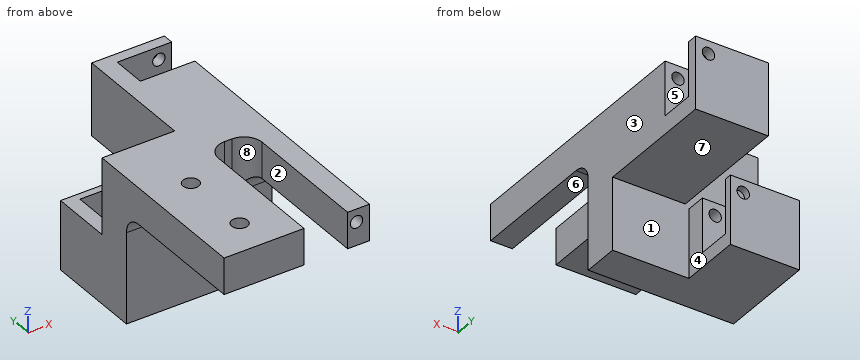
```python
from build123d import *

# Parameters (mm, degrees)
SKETCH1_W               = 40
SKETCH1_H               = 50
BOSS_EXTRUDE1_DEPTH     = 10
SKETCH2_W               = 40
SKETCH2_H               = 10
BOSS_EXTRUDE2_DEPTH     = 30
SKETCH3_W               = 20
SKETCH3_H               = 20
BOSS_EXTRUDE3_DEPTH     = 34
SKETCH4_W               = 19
SKETCH4_H               = 19
BOSS_EXTRUDE4_DEPTH     = 17
CUT_EXTRUDE4_DEPTH      = 9.5
CUT_EXTRUDE13_DEPTH     = 9.5
CUT_EXTRUDE7_DEPTH      = 93.694591653
CUT_EXTRUDE7_DEPTH_BACK = 3
SKETCH10_R              = 1.7
CUT_EXTRUDE9_REACH      = 74.328
SKETCH12_W              = 12
SKETCH12_H              = 40
FILLET2_R               = 5
CUT_EXTRUDE10_REACH     = 74.328
SKETCH13_R              = 2.2
SKETCH14_R              = 1.7
CUT_EXTRUDE14_DEPTH     = 20


with BuildPart() as part:
    # Sketch1 → Boss-Extrude1 (new body)
    with BuildSketch(Plane.XY):
        with Locations((13.634614932, -25)):
            Rectangle(SKETCH1_W, SKETCH1_H)
    extrude(amount=BOSS_EXTRUDE1_DEPTH)

    # Sketch2 → Boss-Extrude2 (add)
    with BuildSketch(Plane.XY):
        with Locations((13.634614932, -5)):
            Rectangle(SKETCH2_W, SKETCH2_H)
    extrude(amount=-BOSS_EXTRUDE2_DEPTH)

    # Sketch3 → Boss-Extrude3 (add)
    with BuildSketch(Plane(origin=(0, 0, 0), x_dir=(1, 0, 0), z_dir=(0, 1, 0))):
        with Locations((23.634614932, 0)):
            Rectangle(SKETCH3_W, SKETCH3_H)
    extrude(amount=BOSS_EXTRUDE3_DEPTH)

    # Sketch4 → Boss-Extrude4 (add)
    with BuildSketch(Plane(origin=(0, 0, 0), x_dir=(1, 0, 0), z_dir=(0, 1, 0))):
        with Locations((3.134614932, 20.5)):
            Rectangle(SKETCH4_W, SKETCH4_H)
    extrude(amount=BOSS_EXTRUDE4_DEPTH)

    # Sketch6 → Cut-Extrude4 (cut)
    with BuildSketch(Plane(origin=(0, 31, 0), x_dir=(1, 0, 0), z_dir=(0, 1, 0))):
        with BuildLine():
            Line((33.634614932, 5), (33.634614932, -10))
            Line((33.634614932, -10), (18.634614932, -10))
            ThreePointArc((18.634614932, -10), (23.028013215, 0.606601718), (33.634614932, 5))
        make_face()
    extrude(amount=-CUT_EXTRUDE4_DEPTH, mode=Mode.SUBTRACT)

    # Sketch7 → Cut-Extrude13 (cut)
    with BuildSketch(Plane(origin=(0, 15, 0), x_dir=(1, 0, 0), z_dir=(0, 1, 0))):
        with BuildLine():
            Line((-2.365385068, 11), (12.634614932, 11))
            Line((12.634614932, 11), (12.634614932, 26))
            ThreePointArc((12.634614932, 26), (2.028013215, 21.606601718), (-2.365385068, 11))
        make_face()
    extrude(amount=-CUT_EXTRUDE13_DEPTH, mode=Mode.SUBTRACT)

    # Sketch10 → Cut-Extrude7 (cut, two sides: drawn at the far end of the back side and taken through both)
    with BuildSketch(Plane(origin=(0, 31, 0), x_dir=(-1, 0, 0), z_dir=(0, -1, 0)).offset(-CUT_EXTRUDE7_DEPTH_BACK)):
        with Locations(Location((-30.099081026, -6.464466094, 0), (0, 0, 180))):
            Circle(SKETCH10_R)
    extrude(amount=CUT_EXTRUDE7_DEPTH + CUT_EXTRUDE7_DEPTH_BACK, mode=Mode.SUBTRACT)

    # Sketch12 → Cut-Extrude9 (cut, up to next)
    with BuildSketch(Plane.XY.offset(10), mode=Mode.PRIVATE) as cut_extrude9_sk1:
        with Locations((21.634614932, -30)):
            Rectangle(SKETCH12_W, SKETCH12_H)
    cut_extrude9_tool1 = extrude(cut_extrude9_sk1.sketch, amount=-CUT_EXTRUDE9_REACH, mode=Mode.PRIVATE) & part.part
    add(cut_extrude9_tool1.solids().sort_by_distance((21.634615, -30, 10))[0], mode=Mode.SUBTRACT)

    # Fillet2
    fillet2_edges = [part.edges().sort_by_distance(p)[0] for p in [
        (4.634614932, -10, 0),
        (30.634614932, -10, 0),
        (27.634614932, -10, 5),
        (15.634614932, -10, 5),
    ]]
    fillet(fillet2_edges, radius=FILLET2_R)

    # Sketch13 → Cut-Extrude10 (cut, up to next)
    with BuildSketch(Plane.XY.offset(10), mode=Mode.PRIVATE) as cut_extrude10_sk1:
        with Locations((4.634614932, -20)):
            Circle(SKETCH13_R)
    cut_extrude10_tool1 = extrude(cut_extrude10_sk1.sketch, amount=-CUT_EXTRUDE10_REACH, mode=Mode.PRIVATE) & part.part
    # Sketch13 → Cut-Extrude10 (cut, up to next)
    with BuildSketch(Plane.XY.offset(10), mode=Mode.PRIVATE) as cut_extrude10_sk2:
        with Locations((4.634614932, -40)):
            Circle(SKETCH13_R)
    cut_extrude10_tool2 = extrude(cut_extrude10_sk2.sketch, amount=-CUT_EXTRUDE10_REACH, mode=Mode.PRIVATE) & part.part
    add(cut_extrude10_tool1.solids().sort_by_distance((4.634615, -20, 10))[0], mode=Mode.SUBTRACT)
    add(cut_extrude10_tool2.solids().sort_by_distance((4.634615, -40, 10))[0], mode=Mode.SUBTRACT)

    # Sketch14 → Cut-Extrude14 (cut)
    with BuildSketch(Plane(origin=(0, 17, 0), x_dir=(1, 0, 0), z_dir=(0, 1, 0))):
        with Locations(Location((9.099081026, 14.535533906, 0), (0, 0, 180))):
            Circle(SKETCH14_R)
    extrude(amount=-CUT_EXTRUDE14_DEPTH, mode=Mode.SUBTRACT)


solid = part.part
```
The model under review builds one solid part; all positions refer to its coordinate system, in mm. Face numbers are marked on the shaded views. A direction names the side the tool comes from. Coordinates: 2 decimals unless noted, no trailing zeros. Order: outer loops, then holes, each group sorted by start corner. A loop starts at its lowest first (then second) coordinate and runs counter-clockwise, first axis right, second up. Notation, with made-up numbers: (-33.5, 74) -> (23.5, 74) arc R25 cw to (23.5, 97) -> close; hole circle Ø2 at (26, 59.25). An arc over 180 degrees is marked (long way). Answer in a Markdown table with one row per item. Add a question column.
Item 1: We need section B-B on y = -20. Write out the cut boundary in (x, z).
Item 2: To check wall thickness, follow probe 1 along X at (y, z) = (-27, 5.5); probe 2 along Y at (x, z) = (10, -24.5); probe 3 along Y at (x, z) = (28.5, 8). State the ranges of each line that lie inside material, in increasing order.
Item 3: We need section A-A on y = -34. Write out the cut boundary in (x, z).
Item 4: We need section C-C on x = 9.5. Write out the cut boundary in (y, z), plus the area to 3 significant figures.
Item 5: We need section D-D on z = 2.5. Write out the cut boundary in (x, y).
Item 6: Clearance check with flat-ended pins moving along their axes: pin 1 (5.5 mm diameter, centred on x = -1, z = -19.5, fed in from +Y); pin 2 (10 mm diameter, centred on x = 13, y = -36.5, fed in from -Z); pin 3 (2.5 mm diameter, centred on x = 9, z = -14.5, fed in from +Y); pin 4 (3.5 mm diameter, centred on x = 4.63, y = -20, fed in from +Z). State where each tip first meets the part, or that it passes through.
Item 7: Mouldability with a two-part tool opening along X and no side actions: class the marked faces 1, 2 and 3 as +X half, -X half, draft (parallel to the pull), parting line (faces both ways), or undercut.
Item 8: Machinability: for the marked faces 4, 5, 6, 7 and 8, which of the approach directions +Z, -Z, +X, -X, +Y, -Y give a long, thin tool a straight path to every point of the face, cutting with its end or side? Answer none if there is none.
Final values:
| question | item | result |
|---|---|---|
| 1 | outline | (-6.37, 0) -> (2.43, 0) -> (2.43, 10) -> (-6.37, 10) -> close; (6.83, 0) -> (15.63, 0) -> (15.63, 10) -> (6.83, 10) -> close; (27.63, 0) -> (33.63, 0) -> (33.63, 10) -> (27.63, 10) -> close; hole circle Ø3.4 at (30.1, 6.46) |
| 2 | probe 1 | x = -6.37 to 15.63, 27.63 to 28.7, 31.5 to 33.63 |
| 2 | probe 2 | y = -10 to 5.5, 15 to 17 |
| 2 | probe 3 | y = -50 to 21.5, 31 to 34 |
| 3 | outline | (-6.37, 0) -> (15.63, 0) -> (15.63, 10) -> (-6.37, 10) -> close; (27.63, 0) -> (33.63, 0) -> (33.63, 10) -> (27.63, 10) -> close; hole circle Ø3.4 at (30.1, 6.46) |
| 4 | outline | (-50, 0) -> (-15, 0) arc R5 cw to (-10, -5) -> (-10, -30) -> (17, -30) -> (17, -16.19) -> (15, -16.19) -> (15, -25.67) -> (5.5, -25.67) -> (5.5, -16.19) -> (-3, -16.19) -> (-3, -12.88) -> (5.5, -12.88) -> (5.5, -11) -> (0, -11) -> (0, 10) -> (-50, 10) -> close; (15, -12.88) -> (17, -12.88) -> (17, -11) -> (15, -11) -> close |
| 4 | area | 954 mm2 |
| 5 | outline | (-6.37, -50) -> (15.63, -50) -> (15.63, -15) arc R5 cw to (20.63, -10) -> (22.63, -10) arc R5 cw to (27.63, -15) -> (27.63, -50) -> (33.63, -50) -> (33.63, 21.5) -> (20.64, 21.5) -> (20.64, 31) -> (33.63, 31) -> (33.63, 34) -> (13.63, 34) -> (13.63, 0) -> (-6.37, 0) -> close; hole circle Ø4.4 at (4.63, -40); hole circle Ø4.4 at (4.63, -20) |
| 6 | pin 1 | stops at y = 17 |
| 6 | pin 2 | stops at z = 0 |
| 6 | pin 3 | stops at y = -3 |
| 6 | pin 4 | passes through |
| 7 | face 1 | draft |
| 7 | face 2 | undercut |
| 7 | face 3 | +X half |
| 8 | face 4 | +Z, -Z, +X, +Y |
| 8 | face 5 | +Z, +X |
| 8 | face 6 | -Z, +X, -X, -Y |
| 8 | face 7 | -Z, +X, -X, +Y |
| 8 | face 8 | +Z, -Z, -Y |
